Input: dimensioned drawing with shaded views. Units: mm. Origin: part minimum x, y, z. A direction names the side the tool comes from. Coordinates: 2 decimals unless noted, no trailing zeros. Order: outer loops, then holes, each group sorted by start corner. A loop starts at its lowest first (then second) coordinate and runs counter-clockwise, first axis right, second up.
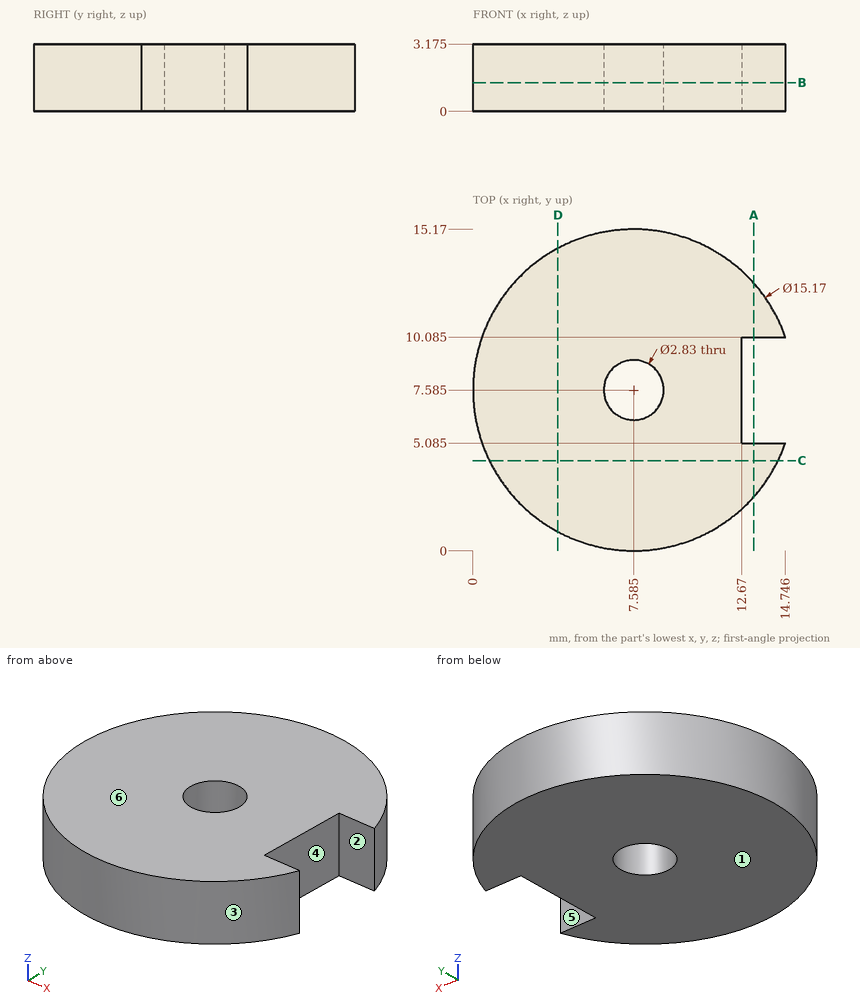
1. Draft query along Y for the marked faces 1, 2, 3 and 4. Return one class per face: released by +Y, released by -Y, zero draft, split by the parting line, or undercut.
Findings:
face 1: zero draft
face 2: undercut
face 3: split by the parting line
face 4: undercut
2. Ray query, line 1 (Y direction, x = 7, z = 2.8); line 2 (X direction, y = 6.75, z = 2.6); line 3 (Y direction, x = 6.5, z = 1.25). Return the intervals inside material, ascending.
Findings:
line 1: y = 0.02 to 6.3, 8.87 to 15.15
line 2: x = 0.05 to 6.44, 8.73 to 12.67
line 3: y = 0.08 to 6.68, 8.49 to 15.09
3. Section query A-A on x = 13.25. Return loops of the section in (y, z) (1 decimal).
Findings:
outline: (2.5, 0) - (5.1, 0) - (5.1, 3.2) - (2.5, 3.2) - close; (10.1, 0) - (12.6, 0) - (12.6, 3.2) - (10.1, 3.2) - close
4. Section query C-C on y = 4.25. Return loops of the section in (x, z) (1 decimal).
Findings:
outline: (0.8, 0) - (14.4, 0) - (14.4, 3.2) - (0.8, 3.2) - close
5. Section query D-D on x = 4. Return loops of the section in (y, z) (1 decimal).
Findings:
outline: (0.9, 0) - (14.3, 0) - (14.3, 3.2) - (0.9, 3.2) - close
6. Pin query (flat end, axial travel): P1, Ø1, axis at y = 3.5, z = 2.5, coming from the -X side; P2, Ø3.5, axis at x = 7.585, y = 7.585, coming from the -Z side; P3, Ø1, axis at x = 14, z = 1.5, coming from the -Y side; P4, Ø1.7, axis at x = 14, z = 1, coming from the +Y side. Return the tip coordinate at first contact, or that it passes through.
Findings:
P1: stops at x = 0.9
P2: stops at z = 0
P3: stops at y = 2.84
P4: stops at y = 12.74
7. Section query B-B on z = 1.35. Return loops of the section in (x, y) (3 decimals).
Findings:
outline: (12.67, 5.085) - (12.67, 10.085) - (14.746, 10.085) arc R7.585 ccw (long way) to (14.746, 5.085) - close; hole circle Ø2.83 at (7.585, 7.585)
8. Access query for the marked faces 5 and 6. Directions: +Z, -Z, +X, -X, +Y, -Y. A direction counts if a zero-diameter tool reaches every point of the face in a straight line with its end or side. Return the directions, or none.
Findings:
face 5: +Z, -Z, +X
face 6: +Z, +X, -X, +Y, -Y
